from build123d import *

# Parameters (mm, degrees)
SKETCH1_R           = 19
BOSS_EXTRUDE1_DEPTH = 10
SKETCH2_R           = 10
CUT_EXTRUDE1_DEPTH  = 2
FILLET1_R           = 1


with BuildPart() as part:
    # Sketch1 → Boss-Extrude1 (new body)
    with BuildSketch(Plane.XY):
        Circle(SKETCH1_R)
    extrude(amount=BOSS_EXTRUDE1_DEPTH)

    # Sketch2 → Cut-Extrude1 (cut)
    with BuildSketch(Plane.XY.offset(10)):
        Circle(SKETCH2_R)
    extrude(amount=-CUT_EXTRUDE1_DEPTH, mode=Mode.SUBTRACT)

    # Fillet1
    fillet1_edges = [part.edges().sort_by_distance(p)[0] for p in [
        (-19, 0, 10),
        (-10, 0, 8),
        (-10, 0, 10),
    ]]
    fillet(fillet1_edges, radius=FILLET1_R - 0.0001)  # a hair under: the kernel refuses the full size


solid = part.part
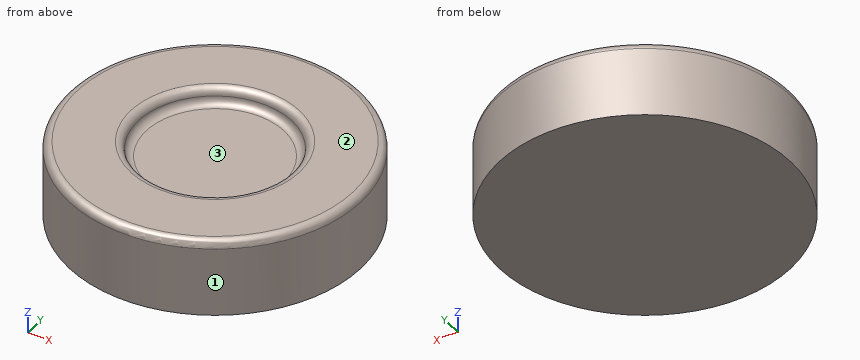
Model file for the job. Use its own axes, mm. Face numbers are marked on the shaded views. Coordinates: 2 decimals unless noted, no trailing zeros. Write each loop counter-clockwise with the first axis right and the second up, starting at its lowest first coordinate (ties: lowest second). Pieces come first, ordered by that corner, then holes. Notation, with made-up numbers: (64, -7.75) -> (110, -7.75) arc R25 cw to (110, 8.25) -> close; hole circle Ø8 at (61, 21.5). An arc over 180 degrees is marked (long way). One line per item, written item: value. Start each with the question number.
1) Slice it at C-C on z = 2. Write the cut outline in (x, y), then the cut area to 3 significant figures.
2) Flat gauge pins, fed straight in: pin 1 Ø12 at (x, y) = (9, -6) entering from -Z; pin 2 Ø4 at (y, z) = (-11, 3) entering from -X; pin 3 Ø2 at (x, z) = (-5, 2) entering from +Y; pin 4 Ø12 at (x, y) = (0, 0) entering from +Z. Where does each tip first touch, or does it go through?
3) Slice it at D-D on z = 8.5. Write the cut outline in (x, y), then the cut area to 3 significant figures.
4) Pull direction Y, two halves, no side cores. Call the marked faces 1, 2 and 3: +Y half, -Y half, draft (parallel to the pull), parting line (faces both ways), or undercut.
5) Probe probe 1 along Y at (x, z) = (0, 9); probe 2 along Z at (x, y) = (-2, 7.5); probe 3 along X at (y, z) = (-7.5, 8.75). List the from-to ranges inside material, lowest first.
Answers follow:
1. outline: circle Ø38 at (0, 0)
1. area: 1,130 mm2
2. pin 1: z = 0
2. pin 2: x = -16.73
2. pin 3: y = 18.57
2. pin 4: z = 8
3. outline: circle Ø38 at (0, 0); hole circle Ø19.73 at (0, 0)
3. area: 828 mm2
4. face 1: parting line
4. face 2: draft
4. face 3: undercut
5. probe 1: -19 to -10, 10 to 19
5. probe 2: 0 to 8
5. probe 3: -17.46 to -6.57, 6.57 to 17.46
